Part model, mm, in its own coordinate system. Round coordinates to 2 decimals unless told otherwise and drop trailing zeros. Write each loop counter-clockwise with the first axis right and the second up, starting at its lowest first coordinate (ties: lowest second). Pieces come first, ordered by that corner, then holes.
1) Saw through at A-A on z = 0. Write the cut outline in (x, y), and give its area (3 significant figures).
2) Saw through at C-C on x = 1.75. Write the cut outline in (y, z).
3) Pull direction Z, two halves, no side cores. Call faces 1 (the flat face through (2.465, 39.44, 4.35)), 2 (the cylindrical face through (-3, 2, 0)), 3 (the flat face through (0, 5, 0)), 4 (the flat face through (-2.465, 39.44, -4.35)): +Z half, -Z half, draft (parallel to the pull), parting line (faces both ways), or undercut.
4) Drill centre lines: L1, parallel to Z at x = 0, y = 1.35; L2, parallel to Y at x = 0, z = 0.25; L3, parallel to Z at x = -1, y = 51.5. Where is each one in solid material? Low to high.
5) Flat gauge pins, fed straight in: pin 1 (3 mm diameter, centred on x = 3, y = 43, fed in from -Z); pin 2 (2 mm diameter, centred on x = -2, y = 23, fed in from -Z); pin 3 (1 mm diameter, centred on x = -2.5, y = 12.5, fed in from +Z). Where does each tip first touch, or does it go through?
6) Saw through at B-B on y = 74.5. Write the cut outline in (x, z), and give its area (3 significant figures).
7) Saw through at D-D on z = -4. Write the cut outline in (x, y), and give its area (3 significant figures).
```python
from build123d import *

# Parameters (mm, degrees)
BOSS_EXTRUDE1_DEPTH = 80
SKETCH2_R           = 3
CUT_EXTRUDE1_DEPTH  = 5


with BuildPart() as part:
    # Sketch1 → Boss-Extrude1 (new body)
    with BuildSketch(Plane(origin=(0, 0, 0), x_dir=(1, 0, 0), z_dir=(0, 1, 0))):
        Polygon((0, 5.773502692), (-5, 2.886751346), (-5, -2.886751346), (0, -5.773502692), (5, -2.886751346), (5, 2.886751346), align=None)
    extrude(amount=BOSS_EXTRUDE1_DEPTH)

    # Sketch2 → Cut-Extrude1 (cut)
    with BuildSketch(Plane.XZ):
        Circle(SKETCH2_R)
    extrude(amount=-CUT_EXTRUDE1_DEPTH, mode=Mode.SUBTRACT)


solid = part.part
```
Completed:
1. outline: (-5, 0) - (-3, 0) - (-3, 5) - (3, 5) - (3, 0) - (5, 0) - (5, 80) - (-5, 80) - close
1. area: 770 mm2
2. outline: (0, -4.76) - (80, -4.76) - (80, 4.76) - (0, 4.76) - (0, 2.44) - (5, 2.44) - (5, -2.44) - (0, -2.44) - close
3. face 1: +Z half
3. face 2: undercut
3. face 3: undercut
3. face 4: -Z half
4. L1: z = -5.77 to -3, 3 to 5.77
4. L2: y = 5 to 80
4. L3: z = -5.2 to 5.2
5. pin 1: stops at z = -4.91
5. pin 2: stops at z = -5.2
5. pin 3: stops at z = 4.62
6. outline: (-5, -2.89) - (0, -5.77) - (5, -2.89) - (5, 2.89) - (0, 5.77) - (-5, 2.89) - close
6. area: 86.6 mm2
7. outline: (-3.07, 0) - (3.07, 0) - (3.07, 80) - (-3.07, 80) - close
7. area: 491 mm2
